The model under review builds one solid part; all positions refer to its coordinate system, in mm. Face numbers are marked on the shaded views. Round coordinates to 2 decimals unless told otherwise and drop trailing zeros. Order: outer loops, then holes, each group sorted by start corner. A loop starts at its lowest first (then second) coordinate and runs counter-clockwise, first axis right, second up. Notation, with made-up numbers: (52, -26.75) -> (58, -26.75) arc R28 cw to (58, 2.25) -> close; hole circle Ø3 at (-28, -18.5). An arc over 180 degrees is marked (long way). Put each result on its own line as item: value. Start each with the question number.
from build123d import *

# Parameters (mm, degrees)
PAD_DEPTH = 30


with BuildPart() as part:
    # Sketch → Pad (new body)
    with BuildSketch(Plane.XZ):
        Polygon((0, 0), (-38, 0), (-38, 18), (-33, 18), (-33, 28), (-38, 28), (-38, 45), (-28, 45), (-2.5, 22), (-2.5, 18), (0, 18), (2.5, 18), (2.5, 22), (28, 45), (38, 45), (38, 28), (33, 28), (33, 18), (38, 18), (38, 0), align=None)
    extrude(amount=PAD_DEPTH)


solid = part.part
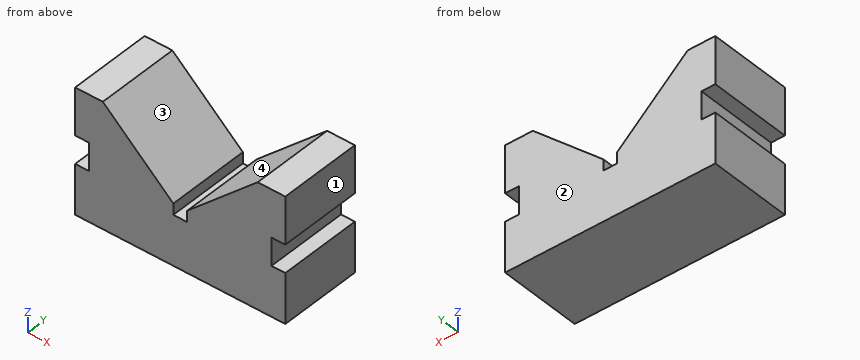
Q1. Take a section at A-A on y = -26. Give the boundary of the cut face in (x, z).
Q2. Draft analysis for pull direction X (two halves, no side actions). For the marked faces 1, 2, 3 and 4, state which applies: +X half, -X half, draft (parallel to the pull), parting line (faces both ways), or undercut.
Q3. Take a section at D-D on x = 17. Give the boundary of the cut face in (y, z), and give its area (3 significant figures).
Q4. Wall thickness on probe 1 along X at (y, z) = (-26.5, 21); probe 2 along X at (y, z) = (-2, 24); probe 3 along Z at (x, y) = (-34, -26): over which ranges is each line inside the solid? List them lowest first. Write a range as [from, to].
Q5. Take a section at C-C on x = 4.5. Give the boundary of the cut face in (y, z).
Q6. Clearance check with flat-ended pins moving along their axes: pin 1 Ø3 at (y, z) = (-7.5, 23) entering from -X; pin 2 Ø5.5 at (x, y) = (0, -20.5) entering from +Z; pin 3 Ø1 at (y, z) = (-14.5, 23) entering from +X. State where each tip first meets the part, or that it passes through.
Q7. Take a section at B-B on z = 36. Give the boundary of the cut face in (x, y).
Calculated:
1. outline: (-38, 0) -> (38, 0) -> (38, 18) -> (33, 18) -> (33, 28) -> (38, 28) -> (38, 45) -> (28, 45) -> (2.5, 22) -> (2.5, 18) -> (-2.5, 18) -> (-2.5, 22) -> (-28, 45) -> (-38, 45) -> (-38, 28) -> (-33, 28) -> (-33, 18) -> (-38, 18) -> close
2. face 1: +X half
2. face 2: draft
2. face 3: undercut
2. face 4: undercut
3. outline: (-30, 0) -> (0, 0) -> (0, 35.08) -> (-30, 35.08) -> close
3. area: 1,050 mm²
4. probe 1: x = [-33, -2.5], [2.5, 33]
4. probe 2: x = [-33, -4.72], [4.72, 33]
4. probe 3: z = [0, 18], [28, 45]
5. outline: (-30, 0) -> (0, 0) -> (0, 23.8) -> (-30, 23.8) -> close
6. pin 1: stops at x = -33
6. pin 2: stops at z = 22.23
6. pin 3: stops at x = 33
7. outline: (-38, -30) -> (-18.02, -30) -> (-18.02, 0) -> (-38, 0) -> close; (18.02, -30) -> (38, -30) -> (38, 0) -> (18.02, 0) -> close
